Build history of the part. All positions in model axes, mm. Face numbers are marked on the shaded views. A direction names the side the tool comes from. Coordinates: 2 decimals unless noted, no trailing zeros. Write each loop counter-clockwise with the first axis right and the second up, starting at its lowest first coordinate (ties: lowest second). Pieces come first, ordered by that corner, then holes. Notation, with made-up numbers: (38.25, 35.25) -> (59.25, 35.25) arc R20 cw to (59.25, 43.25) -> close; hole circle Ø11 at (44.25, 21.5). An arc over 180 degrees is marked (long way). Write each question's results on one line, items separated by ' | '. Start each with the question number.
Q1. Saw through at A-A on y = -8. Give the cut face in (x, z).
Q2. Tool access for the marked faces 1 and 2: list every direction of +Z, -Z, +X, -X, +Y, -Y with a clear straight run to the whole face (end or side of a thin tool).
Q3. Drop a flat-ended pin along its axis: pin 1 Ø0.8 at (y, z) = (-25.5, -0.5) entering from +X. Give the stop position or say it passes through.
Q4. Drill centre lines: line 1 (Z direction, x = -32, y = -50.5); line 2 (X direction, y = 75.5, z = -71.5). Where is each one in solid material? Low to high.
Q5. Saw through at D-D on y = -55.5. Give the cut face in (x, z), and give its area (3 significant figures).
Q6. Saw through at B-B on x = -24.5. Give the cut face in (y, z).
Q7. Saw through at C-C on z = -40.5. Give the cut face in (x, y), and give its area (3 significant figures).
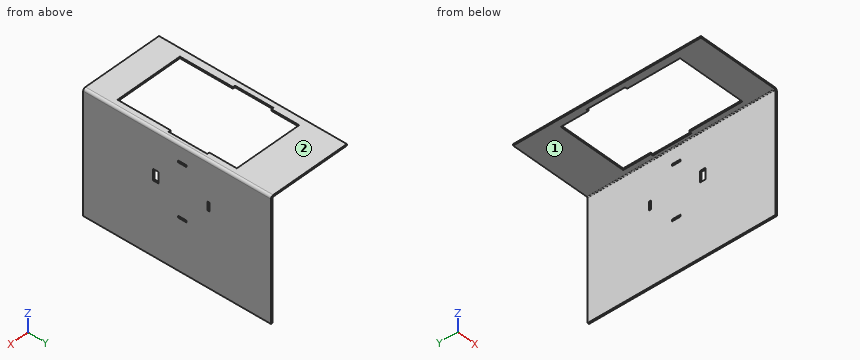
from build123d import *

# Parameters (mm, degrees)
SKETCH1_W                    = 75.36
SKETCH1_H                    = 170
BASE_FLANGE1_DEPTH           = 1.5
EDGE_FLANGE1_STRIP_W         = 7.4732
EDGE_FLANGE1_STRIP_H         = 1.5
EDGE_FLANGE1_STRIP_CUT_DEPTH = 170
EDGE_FLANGE1_DEPTH           = 170
SKETCH11_W                   = 1.7
SKETCH11_H                   = 7.7
SKETCH11_W_2                 = 7.7
SKETCH11_H_2                 = 1.7
SKETCH11_W_3                 = 10
SKETCH11_H_3                 = 5
CUT_EXTRUDE2_DEPTH           = 2


# Sheet-metal steps are written as plain solids
with BuildPart() as part:
    # Sketch1 → Base-Flange1 (new body)
    with BuildSketch(Plane.XY):
        Rectangle(SKETCH1_W, SKETCH1_H)
        Polygon((-31, 23), (-31, 48), (31, 48), (31, 23), (33, 23), (33, -12), (31, -12), (31, -60), (-31, -60), (-31, -12), (-33, -12), (-33, 23), align=None, mode=Mode.SUBTRACT)
    extrude(amount=-BASE_FLANGE1_DEPTH)

    # Edge-Flange1 strip (across the edge) → Edge-Flange1 strip cut (cut)
    with BuildSketch(Plane(origin=(37.68, 85, -1.5), x_dir=(-1, 0, 0), z_dir=(0, -1, 0))):
        with Locations((-1.5, -0.75)):
            Rectangle(EDGE_FLANGE1_STRIP_W, EDGE_FLANGE1_STRIP_H)
    extrude(amount=EDGE_FLANGE1_STRIP_CUT_DEPTH, mode=Mode.SUBTRACT)

    # Edge-Flange1 section (across the edge) → Edge-Flange1 (add)
    with BuildSketch(Plane(origin=(37.68, 85, -1.5), x_dir=(-1, 0, 0), z_dir=(0, -1, 0))):
        with BuildLine():
            Line((0, 0.7366), (0, 108.5))
            Line((0, 108.5), (1.5, 108.5))
            Line((1.5, 108.5), (1.5, 0.7366))
            ThreePointArc((1.5, 0.7366), (1.715745145, 0.215745145), (2.2366, 0))
            Line((2.2366, 0), (2.2366, -1.5))
            ThreePointArc((2.2366, -1.5), (0.655084973, -0.844915027), (0, 0.7366))
        make_face()
    extrude(amount=EDGE_FLANGE1_DEPTH)

    # Sketch11 → Cut-Extrude2 (cut)
    with BuildSketch(Plane(origin=(37.68, 0, 0), x_dir=(0, 0, -1), z_dir=(1, 0, 0))):
        with Locations((63.463831766, 4.61334704)):
            Rectangle(SKETCH11_W, SKETCH11_H)
        with Locations((39.613831766, 28.46334704)):
            Rectangle(SKETCH11_W_2, SKETCH11_H_2)
        with Locations((15.763831766, 4.61334704)):
            Rectangle(SKETCH11_W, SKETCH11_H)
        with Locations((39.613831766, -19.23665296)):
            Rectangle(SKETCH11_W_3, SKETCH11_H_3)
    extrude(amount=-CUT_EXTRUDE2_DEPTH, mode=Mode.SUBTRACT)


solid = part.part
Returned:
1) outline: (-37.68, -1.5) -> (-33, -1.5) -> (-33, 0) -> (-37.68, 0) -> close; (33, -1.5) -> (35.44, -1.5) arc R0.74 cw to (36.18, -2.24) -> (36.18, -110) -> (37.68, -110) -> (37.68, -2.24) arc R2.24 ccw to (35.44, 0) -> (33, 0) -> close
2) face 1: -Z, -X, +Y, -Y | face 2: +Z, +X, -X, +Y, -Y
3) pin 1: stops at x = 37.24
4) line 1: z = -1.5 to 0 | line 2: x = 36.18 to 37.68
5) outline: (-37.68, -1.5) -> (-31, -1.5) -> (-31, 0) -> (-37.68, 0) -> close; (31, -1.5) -> (35.44, -1.5) arc R0.74 cw to (36.18, -2.24) -> (36.18, -110) -> (37.68, -110) -> (37.68, -2.24) arc R2.24 ccw to (35.44, 0) -> (31, 0) -> close | area: 182 mm2
6) outline: (-85, -1.5) -> (-60, -1.5) -> (-60, 0) -> (-85, 0) -> close; (48, -1.5) -> (85, -1.5) -> (85, 0) -> (48, 0) -> close
7) outline: (36.18, -85) -> (37.68, -85) -> (37.68, -21.74) -> (36.18, -21.74) -> close; (36.18, -16.74) -> (37.68, -16.74) -> (37.68, 27.61) -> (36.18, 27.61) -> close; (36.18, 29.31) -> (37.68, 29.31) -> (37.68, 85) -> (36.18, 85) -> close | area: 245 mm2
